from build123d import *

# Parameters (mm, degrees)
F0_W     = 90.9828
F0_H     = 4.3688
F0_W_2   = 90.17
F0_H_2   = 3.556
F1_DEPTH = 50.8
F2_DEPTH = 0.762
F4_DEPTH = 4.3698


with BuildPart() as f1:
    # F0 (on Top) → F1 (new body)
    with BuildSketch(Plane.XY):
        Rectangle(F0_W, F0_H)
        Rectangle(F0_W_2, F0_H_2, mode=Mode.SUBTRACT)
    extrude(amount=F1_DEPTH)

    # F0 (on Top) → F2 (join)
    with BuildSketch(Plane.XY):
        Rectangle(F0_W, F0_H)
        Rectangle(F0_W_2, F0_H_2, mode=Mode.SUBTRACT)
        Rectangle(F0_W_2, F0_H_2)
    extrude(amount=F2_DEPTH)

    # F3 (on face) → F4 (cut, through all)
    with BuildSketch(Plane.XZ.offset(2.1844)):
        with BuildLine():
            Line((13.7414, 50.8), (-13.7414, 50.8))
            ThreePointArc((-13.7414, 50.8), (0, 37.0586), (13.7414, 50.8))
        make_face()
    extrude(amount=-F4_DEPTH, mode=Mode.SUBTRACT)


solid = f1.part
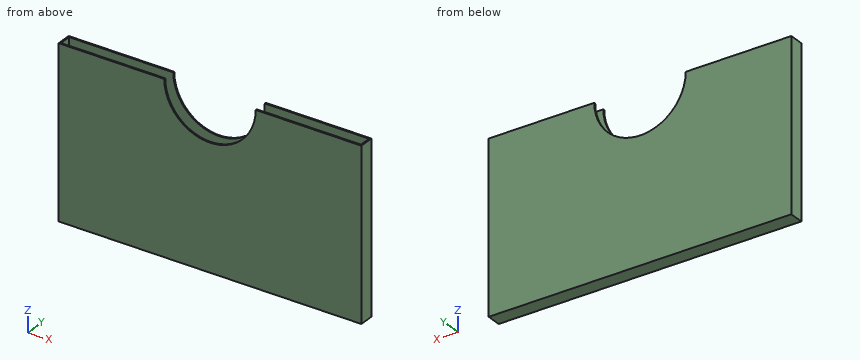
Input: part model. Units: mm. Frame: model coordinates. Coordinates: 2 decimals unless noted, no trailing zeros. Loops run counter-clockwise (first coordinate to the right, second up) from the corner with the lowest first, then second, coordinate; pieces in that order, holes last.
Q1. Material intervals for line 1 (X direction, y = 1.45, z = 22.5) (3 decimals); line 2 (Y direction, x = 21, z = 23.5); line 3 (Z direction, x = 27.5, y = 0.75), sorted ascending.
Q2. Cut plane D-D (z = 45). Output: boundary loops of the cut face in (x, y) (3 decimals).
Q3. Cut plane A-A (z = 6). Output: boundary loops of the cut face in (x, y) (3 decimals), then the cut area to 3 significant figures.
Q4. Cut plane C-C (x = 39.5). Output: boundary loops of the cut face in (y, z).
Q5. Cut plane B-B (y = 0.7). Output: boundary loops of the cut face in (x, z) (3 decimals).
Working result:
1. line 1: x = -45.491 to -45.085, 45.085 to 45.491
1. line 2: y = -2.18 to -1.78, 1.78 to 2.18
1. line 3: z = 0 to 0.76
2. outline: (-45.491, -2.184) - (-12.457, -2.184) - (-12.457, -1.778) - (-45.085, -1.778) - (-45.085, 1.778) - (-12.457, 1.778) - (-12.457, 2.184) - (-45.491, 2.184) - close; (12.457, -2.184) - (45.491, -2.184) - (45.491, 2.184) - (12.457, 2.184) - (12.457, 1.778) - (45.085, 1.778) - (45.085, -1.778) - (12.457, -1.778) - close
3. outline: (-45.491, -2.184) - (45.491, -2.184) - (45.491, 2.184) - (-45.491, 2.184) - close; hole (-45.085, -1.778) - (45.085, -1.778) - (45.085, 1.778) - (-45.085, 1.778) - close
3. area: 76.8 mm2
4. outline: (-2.18, 0) - (2.18, 0) - (2.18, 50.8) - (1.78, 50.8) - (1.78, 0.76) - (-1.78, 0.76) - (-1.78, 50.8) - (-2.18, 50.8) - close
5. outline: (-45.491, 0) - (45.491, 0) - (45.491, 50.8) - (45.085, 50.8) - (45.085, 0.762) - (-45.085, 0.762) - (-45.085, 50.8) - (-45.491, 50.8) - close
